Autodesk Inventor part; units mm, degrees
ref_plane "YZ Plane" through (0, 0, 0) normal (1, 0, 0) x (0, 1, 0)
ref_plane "XZ Plane" through (0, 0, 0) normal (0, 1, 0) x (-1, 0, 0)
ref_plane "XY Plane" through (0, 0, 0) normal (0, 0, 1) x (1, 0, 0)
sketch "Náčrt1" plane through (0, 0, 0) normal (0, 1, 0) x (-1, 0, 0)
  line L0 (0, 0) -> (50, 0)
  line L1 (50, 0) -> (66.0697, -19.1511)
  line L2 (50, 0) -> (75, 0) construction
  line L3 (66.0697, -19.1511) -> (58.4092, -25.579)
  line L4 (0, -12) -> (0, 0)
  line L5 (58.6554, -25.3724) -> (47.4347, -12)
  line L6 (47.4347, -12) -> (0, -12)
  dimension "d0" = 50
  dimension "d2" = 25
  dimension "d3" = 50
  dimension "d4" = 10
  dimension "d5" = 12
extrude "Vysunutí1" add sketch "Náčrt1" along normal blind 15
sketch "Náčrt11" plane through (0, 0, 0) normal (1, 0, 0) x (0, 0, -1)
  line L0 (0, 0) -> (0, 15)
  line L1 (0, 7.5) -> (12, 7.5)
  line L2 (12, 0) -> (12, 15)
  line L3 (0, 3.5) -> (4, 3.5)
  line L4 (4, 3.5) -> (4, 11.5)
  line L5 (4, 11.5) -> (0, 11.5)
  line L6 (0, 11.5) -> (0, 3.5)
  point P0 (0, 7.5)
  point P1 (0, 11.5)
  dimension "d64" = 4
  dimension "d65" = 8
extrude "Vysunutí10" cut sketch "Náčrt11" against normal through all
sketch "Náčrt21" plane through (-66.0697, 0, -19.1511) normal (-0.6427876, 0, -0.7660444) x (-0.7660444, 0, 0.6427876)
  line L0 (0, 0) -> (0, 15)
  line L1 (0, 3.5) -> (-4, 3.5)
  line L2 (-4, 3.5) -> (-4, 11.5)
  line L3 (-4, 11.5) -> (0, 11.5)
  line L4 (0, 11.5) -> (0, 3.5)
  point P0 (-38.3022, 0)
  point P1 (0, 7.5)
  point P2 (0, 11.5)
  dimension "d68" = 4
  dimension "d69" = 8
extrude "Vysunutí11" cut sketch "Náčrt21" against normal through all
sketch "Náčrt30" plane through (0, 0, -12) normal (0, 0, -1) x (-1, 0, 0)
  point P0 (0, 0)
sketch "Náčrt31" plane through (0, 0, 0) normal (1, 0, 0) x (0, 0, -1)
  point P0 (0, 0)
sketch "Náčrt32" plane through (0, 0, 0) normal (0, -1, 0) x (1, 0, 0)
  line L0 (-47.4347, -12) -> (-58.6554, -25.3724)
  line L1 (-47.4347, -12) -> (-47.4347, 0)
  line L2 (-47.4347, -12) -> (-58.6554, -25.3724)
  line L3 (-58.6554, -25.3724) -> (-66.0697, -19.1511)
  line L4 (-66.0697, -19.1511) -> (-50, 0)
  line L5 (-50, 0) -> (-47.4347, 0)
  line L6 (-50, 0) -> (0, 0)
  point P0 (-47.4347, 0)
extrude "Vysunutí16" add sketch "Náčrt32" against normal through all
sketch "Náčrt33" plane through (0, 0, 0) normal (0, -1, 0) x (1, 0, 0)
  line L0 (-47.4347, -12) -> (-58.6554, -25.3724)
  line L1 (-47.4347, -4) -> (-47.4347, 0)
  line L2 (-47.4347, -12) -> (-47.4347, 0)
  line L3 (-66.0697, -19.1511) -> (-50, 0)
  line L4 (-47.4347, 0) -> (-50, 0)
  line L5 (-50, 0) -> (-66.0697, -19.1511)
  line L6 (-50, 0) -> (0, 0)
  line L7 (-66.0697, -19.1511) -> (-50, 0)
  line L8 (-58.6554, -25.3724) -> (-66.0697, -19.1511)
  line L9 (-47.4347, -12) -> (-58.6554, -25.3724)
  line L10 (0, -12) -> (-47.4347, -12)
  line L11 (0, 0) -> (0, -12)
  line L12 (-58.6554, -25.3724) -> (-66.0697, -19.1511)
  line L13 (-66.0697, -19.1511) -> (-58.6554, -25.3724)
  line L14 (-58.6554, -25.3724) -> (-47.4347, -12)
extrude "Vysunutí17" cut sketch "Náčrt33" against normal through all contours L0 L8 L3 L4 L1 L2
sketch "Náčrt34" plane through (0, 0, 0) normal (0, -1, 0) x (1, 0, 0)
  line L0 (-47.4347, 0) -> (-47.4347, -12)
  line L1 (-47.4347, 0) -> (-47.4347, -12)
  line L2 (0, -12) -> (-47.4347, -12)
  line L3 (0, 0) -> (0, -12)
  line L4 (-47.4347, 0) -> (0, 0)
  line L5 (0, -12) -> (-47.4347, -12)
  line L6 (-44, -12) -> (-47.4347, -9.595)
  line L7 (-44, -12) -> (-39.807, -12) construction
  line L8 (-47.4347, -9.595) -> (-47.4347, -12)
  line L9 (-44, -12) -> (-47.4347, -12)
  line L10 (0, 0) -> (-47.4347, 0)
  line L11 (-44, 0) -> (-47.0563, -2.14)
  line L12 (-44, 0) -> (-40.269, 0) construction
  line L13 (-47.0563, -2.14) -> (-47.4347, -2.405)
  line L14 (-47.4347, -2.405) -> (-47.4347, 0)
  line L15 (-44, 0) -> (-47.4347, 0)
  dimension "d99" = 145
  dimension "d100" = 145
extrude "Vysunutí18" cut sketch "Náčrt34" against normal through all contours L4 L11 L13 L0 | L6 L2 L0
sketch "Náčrt39" plane through (0, 0, 0) normal (1, 0, 0) x (0, 0, -1)
  line L0 (0, 11.5) -> (0, 15)
  line L1 (12, 0) -> (12, 15)
  line L2 (0, 0) -> (0, 3.5)
  line L3 (1, 0.75) -> (10, 0.75)
  line L4 (10, 14.25) -> (1, 14.25)
  line L5 (1, 14.25) -> (1, 12.2503)
  line L6 (4, 4.7) -> (4, 10.3)
  line L7 (5, 12.2503) -> (1, 12.2503)
  line L8 (1, 0.75) -> (1, 2.7496)
  line L9 (1, 2.7496) -> (5, 2.7496)
  line L10 (5, 2.7496) -> (5, 12.2503)
  line L11 (10, 0.75) -> (10, 14.25)
  line L12 (4, 7.5) -> (12, 7.5)
  line L13 (12, 9.95) -> (12, 5.05)
  point P0 (1, 1.7498)
  point P1 (5, 7.5)
  point P2 (1, 13.2502)
  point P3 (10, 7.5)
  point P4 (5.5, 0.75)
  dimension "d119" = 13.5
extrude "Vysunutí22" add sketch "Náčrt39" along normal blind 10
sketch "Náčrt40" plane through (0, 0, 0) normal (0, -1, 0) x (1, 0, 0)
  line L0 (-47.4347, -2.405) -> (-47.4347, -9.595)
  line L1 (-47.4347, -6) -> (0, -6)
  line L2 (-44, 0) -> (-47.4347, -2.405)
  line L3 (-47.4347, -2.405) -> (-47.4347, -9.595)
  line L4 (-47.4347, -9.595) -> (-44, -12)
  line L5 (0, -12) -> (-44, -12)
  line L6 (0, 0) -> (0, -12)
  line L7 (-44, 0) -> (0, 0)
  line L8 (-27.885, -6) -> (-22.985, -6)
  line L9 (-25.435, -6) -> (-25.435, 0)
  line L10 (-25.435, -6) -> (-25.435, -12)
  dimension "d124" = 47.4347
extrude "Vysunutí24" cut sketch "Náčrt40" against normal through all contours L2 L7 L9 L1 L0 | L1 L10 L5 L4 L0
sketch "Náčrt41" plane through (0, 15, 0) normal (0, 1, 0) x (1, 0, 0)
  line L0 (-25.435, 0) -> (0, 0)
  line L1 (-25.435, 0) -> (-22, 0)
  line L2 (-22, 0) -> (-25.435, 2.4052)
  line L3 (-25.435, 12) -> (-25.435, 0)
  line L4 (-25.435, 2.4052) -> (-25.435, 0)
  line L5 (-22, 0) -> (-25.435, 0)
  line L6 (0, 12) -> (-25.435, 12)
  line L7 (-22, 12) -> (-17.9846, 12) construction
  line L8 (-25.435, 9.6038) -> (-21.9829, 12)
  line L9 (-25.435, 9.6038) -> (-25.435, 12)
  line L10 (-21.9829, 12) -> (-25.435, 12)
  dimension "d127" = 3.435
  dimension "d128" = 35
extrude "Vysunutí25" cut sketch "Náčrt41" against normal through all
sketch "Náčrt42" plane through (0, 3.5, -4) normal (0, 0, 1) x (1, 0, 0)
  line L0 (-25.435, 8) -> (-25.435, 0)
  line L1 (-25.435, 4) -> (0, 4)
  line L2 (0, -3.5) -> (0, 11.5)
  line L3 (-21.9829, -3.5) -> (-21.9829, 11.5)
  line L4 (-21.9829, 4) -> (-16.0829, 4)
  circle A0 centre (-16.0829, 4) radius 2.9
  line L5 (-13.1829, 4) -> (-10.1829, 4)
  circle A1 centre (-7.3829, 4) radius 2.9
  line L6 (-10.2829, 7.4092) -> (-10.2829, 0.965)
  dimension "d133" = 5.8
  dimension "d132" = 5.9
  dimension "d134" = 3
  dimension "d136" = 5.8
extrude "Vysunutí26" cut sketch "Náčrt42" against normal through all
properties part number "chodecsemafor"
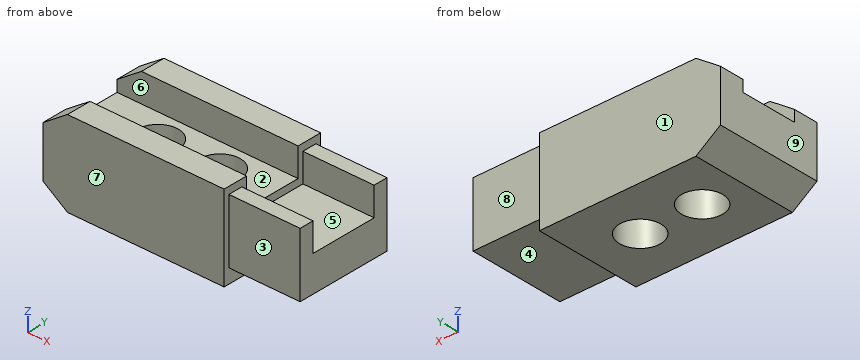
Model file for the job. Use its own axes, mm. Face numbers are marked on the shaded views. A direction names the side the tool comes from. Round coordinates to 2 decimals unless told otherwise and drop trailing zeros. Loops run counter-clockwise (first coordinate to the right, second up) from the corner with the lowest first, then second, coordinate; pieces in that order, holes last. Notation, with made-up numbers: M -39.75,79.25 L -22.75,79.25 A18 ccw -22.75,100.25 Z; hole C -8.5,67.5 d3. An arc over 180 degrees is marked long. Put each result on its own line as item: value. Start each with the question number.
Item 1: 3-axis set-ups, long thin cutter, end or side, ignore diameter. For the marked faces 5, 6, 7, 8 and 9: which of +Z, -Z, +X, -X, +Y, -Y reach the whole face in a straight line?
Item 2: Cut at B-B (y = 7.5). List the corners of the cut face in (x, z) (3 decimals).
Item 3: Drop flat-ended pins along their axis: P1, Ø5, axis at x = -16.08, y = 7.5, coming from the -Z side; P2, Ø2, axis at x = 3.5, z = -7.5, coming from the +Y side; P3, Ø2.5, axis at x = 4.5, z = -6, coming from the -Y side; P4, Ø0.6, axis at x = 4.5, y = 13.5, coming from the +Z side. Give the stop position or say it passes through.
Item 4: Cut at C-C (z = -7.5). List the corners of the cut face in (x, y) (3 decimals).
Item 5: Mould opens along Y. For the marked faces 1, 2, 3 and 4 say: released by +Y, released by -Y, zero draft, split by the parting line, or undercut.
Item 6: Drill centre lines: line 1 along X through (y, z) = (7.5, -7) (3 decimals); line 2 along Y through (x, z) = (-14, -2.5); line 3 along Z through (x, y) = (-3, 8). Where is each one in solid material? Low to high.
Item 7: Cut at D-D (x = 6). List the corners of the cut face in (y, z).
Item 8: Cut at A-A (x = -5). List the corners of the cut face in (y, z), then the cut area to 3 significant figures.
Answer block:
1. face 5: +Z, +X
1. face 6: +Z, +X, -X
1. face 7: +Z, -Z, +X, -X, -Y
1. face 8: +Z, -Z, +X, +Y
1. face 9: +Z, -Z, -X, +Y, -Y
2. outline: M -25.435,-9.604 L -21.983,-12 L -18.983,-12 L -18.983,-4 L -25.435,-4 Z; M -13.183,-12 L -10.283,-12 L -10.283,-4 L -13.183,-4 Z; M -4.483,-12 L 0,-12 L 0,-10 L 10,-10 L 10,-5 L 0,-5 L 0,-4 L -4.483,-4 Z
3. P1: through
3. P2: y = 14.25
3. P3: y = 0.75
3. P4: z = -1
4. outline: M -25.435,0 L 0,0 L 0,0.75 L 10,0.75 L 10,14.25 L 0,14.25 L 0,15 L -25.435,15 Z; hole C -16.083,7.5 d5.8; hole C -7.383,7.5 d5.8
5. face 1: released by +Y
5. face 2: undercut
5. face 3: released by -Y
5. face 4: zero draft
6. line 1: -25.435 to -18.983, -13.183 to -10.283, -4.483 to 10
6. line 2: 0 to 3.5, 11.5 to 15
6. line 3: -12 to -4
7. outline: M 0.75,-10 L 14.25,-10 L 14.25,-1 L 12.25,-1 L 12.25,-5 L 2.75,-5 L 2.75,-1 L 0.75,-1 Z
8. outline: M 0,-12 L 5.85,-12 L 5.85,-4 L 3.5,-4 L 3.5,0 L 0,0 Z; M 9.15,-12 L 15,-12 L 15,0 L 11.5,0 L 11.5,-4 L 9.15,-4 Z
8. area: 122 mm2
